Build history of the part. All positions in model axes, mm. Give positions to 0.01 mm unless a question says otherwise; leave off trailing zeros. Loops run counter-clockwise (first coordinate to the right, second up) from the corner with the lowest first, then second, coordinate; pieces in that order, holes last. Notation, with made-up numbers: (36, 76.5) - (46, 76.5) arc R17 ccw to (46, 95.5) - close; hole circle Ø10 at (5.25, 10). An arc over 180 degrees is marked (long way). Return JSON: item names as keys, results as strings. Group by question number.
1) Slice it at A-A (z = 1.75). Count the separate pieces of the cut face and the enclosed holes in it, and give its area (3 significant figures).
2) Drill centre lines: probe 1 along Y at (x, z) = (-0.5, 3.15); probe 2 along Y at (x, z) = (8.5, 2.95); probe 3 along X at (y, z) = (-22.5, 2.7). Where is each one in solid material? Low to high. Write a range as from..to.
3) Slice it at B-B (y = -35.5). List the corners of the cut face in (x, z), and give its area (3 significant figures).
4) Drop flat-ended pins along their axis: pin 1 (2 mm diameter, centred on y = -11, z = 3.5, fed in from +X); pin 2 (4 mm diameter, centred on x = 7.28, y = 10.4, fed in from +Z); pin 3 (1.5 mm diameter, centred on y = 17.5, z = 3, fed in from +X). Give the stop position or say it passes through.
5) Slice it at C-C (y = 56.5). List the corners of the cut face in (x, z).
Autodesk Inventor part; units mm, degrees
ref_plane "YZ Plane" through (0, 0, 0) normal (1, 0, 0) x (0, 1, 0)
ref_plane "XZ Plane" through (0, 0, 0) normal (0, 1, 0) x (-1, 0, 0)
ref_plane "XY Plane" through (0, 0, 0) normal (0, 0, 1) x (1, 0, 0)
sketch "Sketch1" plane through (0, 0, 0) normal (0, 0, 1) x (1, 0, 0)
  circle A0 centre (0, 0) radius 63.5 construction
  circle A1 centre (0, 0) radius 7.1437
  circle A2 centre (0, 0) radius 12.7 construction
  circle A3 centre (0, 0) radius 19.05
  line L0 (0, 63.5) -> (0, 0) construction
  line L1 (0, 63.5) -> (4.306, 47.4299)
  line L2 (4.306, 47.4299) -> (-16.6992, 9.1674)
  circle A4 centre (0, 0) radius 47.625 construction
  arc A5 (31.8711, 50.0344) -> (0, 63.5) centre (0, 19.05) ccw
  line L3 (31.8711, 50.0344) -> (18.5028, -4.533)
  circle A6 centre (0, 0) radius 44.45 construction
  line L4 (30.03, -32.772) -> (0, 0) construction
  line L5 (30.03, -32.772) -> (19.7345, -24.8719)
  line L6 (19.7345, -24.8719) -> (19.0429, 0.5186)
  circle A7 centre (0, 0) radius 31.75 construction
  arc A8 (-42.3927, -13.3664) -> (30.03, -32.772) centre (0, 0) ccw
  line L7 (-42.3927, -13.3664) -> (-12.9621, 13.9602)
  line L8 (-42.3927, -13.3664) -> (0, 0) construction
  line L9 (-2.2951, 18.9112) -> (10.5685, 42.3434)
  line L10 (14.4751, 12.3844) -> (20.8358, 38.3475)
  arc A9 (20.8358, 38.3475) -> (10.5685, 42.3434) centre (15.4391, 39.6696) ccw
  line L11 (-10.9985, 6.35) -> (0, 0) construction
  line L12 (0, 0) -> (-5.3673, 11.5101) construction
  circle A10 centre (-5.3673, 11.5101) radius 1.7526
  circle A11 centre (-12.6517, 1.1069) radius 1.7526
  circle A12 centre (-7.2844, -10.4032) radius 1.7526
  circle A13 centre (5.3673, -11.5101) radius 1.7526
  circle A14 centre (12.6517, -1.1069) radius 1.7526
  circle A15 centre (7.2844, 10.4032) radius 1.7526
  arc A16 (-15.4432, -20.166) -> (-4.1463, -25.0593) centre (0, 0) ccw construction
  arc A17 (-19.304, -25.2075) -> (-5.1829, -31.3241) centre (0, 0) ccw
  arc A18 (-11.5824, -15.1245) -> (-3.1097, -18.7945) centre (0, 0) ccw
  arc A19 (-11.5824, -15.1245) -> (-19.304, -25.2075) centre (-15.4432, -20.166) ccw
  arc A20 (-5.1829, -31.3241) -> (-3.1097, -18.7945) centre (-4.1463, -25.0593) ccw
  line L13 (-15.4432, -20.166) -> (0, 0) construction
  line L14 (-4.1463, -25.0593) -> (0, 0) construction
  line L15 (0, 0) -> (-10.0957, -23.3074) construction
  point P0 (19.1127, -2.0435)
  point P1 (-15.2178, 11.8657)
  point P2 (-3.1097, -18.7945)
  dimension "d0" = 127
  dimension "d8" = 38.1
  dimension "d14" = 15.875
  dimension "d17" = 63.5
  dimension "d1" = 14.2875
  dimension "d2" = 25.4
  dimension "d9" = 15
  dimension "d11" = 44.45
  dimension "d12" = 15
  dimension "d15" = 88.9
  dimension "d16" = 10
  dimension "d18" = 42.5
  dimension "d19" = 115
  dimension "d28" = 7.9375
  dimension "d29" = 7.9375
  dimension "d30" = 5.5563
  dimension "d31" = 35
  dimension "d32" = 3.5052
  dimension "d35" = 360
  dimension "d40" = 60
  dimension "d41" = 12.7
  dimension "d43" = 28.05
  dimension "d44" = 156.58
extrude "Extrusion1" add sketch "Sketch1" along normal blind 4.7625 contours A3 | A3 L6 L3 | A3 L10 A9 L9 L7 L2 L1 A5 L3 L6 | L3 L6 L5 A8 L7 L2 A3 A19 A17 A20 | A3 L2 L7
fillet "Fillet1" radius 3.175 6 edges at (19.1127, -2.0435, 2.3813) (19.7345, -24.8719, 2.3813) (4.306, 47.4299, 2.3813) (-2.2951, 18.9112, 2.3813) (14.4751, 12.3844, 2.3813) (-15.2178, 11.8657, 2.3813)
fillet "Fillet3" radius 3.175 1 edges at (-42.3927, -13.3664, 2.3813)
sketch "Sketch2" plane through (0, 0, 4.7625) normal (0, 0, 1) x (1, 0, 0)
  arc A0 (31.8711, 50.0344) -> (0, 63.5) centre (0, 19.05) ccw construction
  circle A1 centre (0, 0) radius 63.5 construction
equation "\"d29\" = d28"
properties part number "Blade" material "Steel, Alloy"
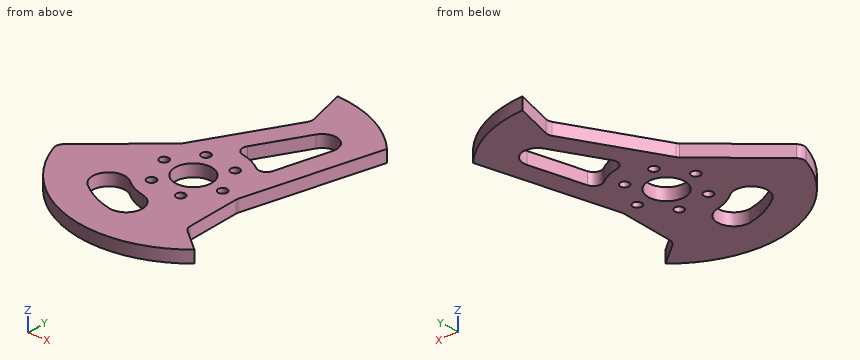
Results:
{
 "1": {"separate pieces": "1", "enclosed holes": "9", "area": "3,470 mm2"},
 "2": {"probe 1": "-44.45..-30.26, -19.86..-7.13, 7.13..38.68", "probe 2": "-43.63..9.14, 11.67..17.05, 38.58..62.68", "probe 3": "-38.33..-21.35, 1.67..19.67"},
 "3": {"outline": "(-26.75, 0) - (26.75, 0) - (26.75, 4.76) - (-26.75, 4.76) - close", "area": "255 mm2"},
 "4": {"pin 1": "x = 19.38", "pin 2": "z = 4.76", "pin 3": "x = 24.08"},
 "5": {"outline": "(1.88, 0) - (23.94, 0) - (23.94, 4.76) - (1.88, 4.76) - close"}
}
